Geometry check sheet. Reference: drawing and pictorial views, mm from the part's lowest x, y, z. A direction names the side the tool comes from. Coordinates: 2 decimals unless noted, no trailing zeros. Loops run counter-clockwise (first coordinate to the right, second up) from the corner with the lowest first, then second, coordinate; pieces in that order, holes last. Notation, with made-up numbers: (67, 89.5) -> (118, 89.5) arc R18 ccw to (118, 116.5) -> close; hole circle Ø6 at (87.25, 82.5). An arc over 180 degrees is marked (long way). Use one line per item in the form item = value.
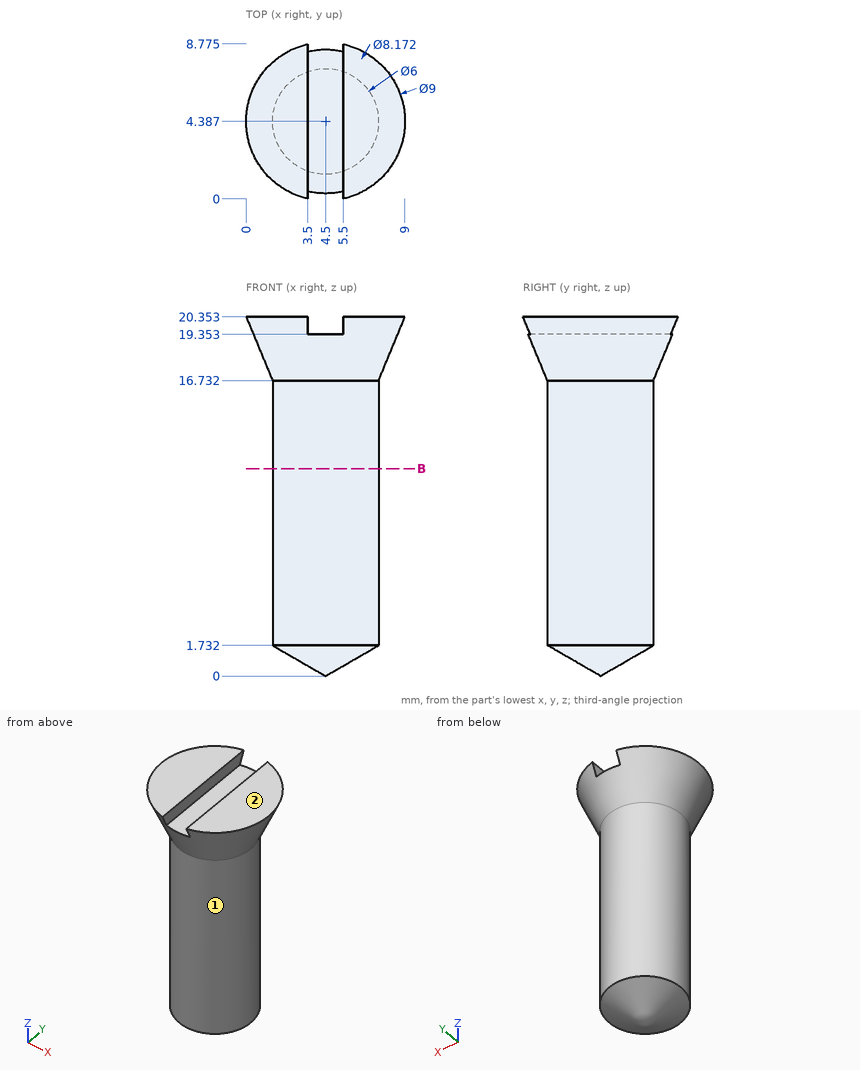
(1) Scan lines: line 1 along Y through (x, z) = (4.5, 14.25); line 2 along Y through (x, z) = (5.5, 15) (1 decimal); line 3 along Z through (x, y) = (7.25, 3.5) (1 decimal). Record each from-to range of solid material in increasing order.
Established:
line_1 = 1.39 to 7.39
line_2 = 1.6 to 7.2
line_3 = 1.7 to 20.4
(2) Tool access check on the marked faces 1 and 2. Record the directions out of +Z, -Z, +X, -X, +Y, -Y that give a thin tool (end or side, any length) a straight path to the whole face; none if there is none.
Established:
face_1 = -Z
face_2 = +Z, +X, -X, +Y, -Y
(3) Section check B-B, the plane z = 11.75. Record the boundary of the cut face in (x, y).
Established:
outline = circle Ø6 at (4.5, 4.39)
(4) Go/stop test with flat-tipped pins: P1, Ø0.5, axis at y = 4, z = 19.5, coming from the +X side (1 decimal); P2, Ø1.5, axis at y = 5, z = 10.5, coming from the +X side; P3, Ø0.6, axis at x = 4.5, y = 5, coming from the +Z side. Record where each tip stops, or that it passes through.
Established:
P1 = 8.7
P2 = 7.5
P3 = 19.35
